from build123d import *

# Parameters (mm, degrees)
EXTRUDE_1_DEPTH     = 8
FILLET_1_R          = 20
SKETCH_5_R          = 10.5
SKETCH_5_R_2        = 6
CUT_EXTRUDE_4_DEPTH = 10
CUT_EXTRUDE_5_DEPTH = 10


with BuildPart() as part:
    # 草图1 → 凸台-拉伸1 (new body)
    with BuildSketch(Plane.XY):
        with BuildLine():
            Line((0, -10), (0, 10))
            Line((0, 10), (11.180339887, 10))
            ThreePointArc((11.180339887, 10), (-15, 0), (11.180339887, -10))
            Line((11.180339887, -10), (0, -10))
        make_face()
        with BuildLine():
            Line((11.180339887, 10), (0, 10))
            Line((0, 10), (0, -10))
            Line((0, -10), (11.180339887, -10))
            ThreePointArc((11.180339887, -10), (14.012585384, -5.352331347), (15, 0))
            ThreePointArc((15, 0), (14.012585384, 5.352331347), (11.180339887, 10))
        make_face()
        with BuildLine():
            Line((188.819660113, 10), (11.180339887, 10))
            ThreePointArc((11.180339887, 10), (14.012585384, 5.352331347), (15, 0))
            ThreePointArc((15, 0), (14.012585384, -5.352331347), (11.180339887, -10))
            Line((11.180339887, -10), (188.819660113, -10))
            ThreePointArc((188.819660113, -10), (185, 0), (188.819660113, 10))
        make_face()
        with BuildLine():
            ThreePointArc((215, 0), (205.352331347, 14.012585384), (188.819660113, 10))
            Line((188.819660113, 10), (200, 10))
            Line((200, 10), (200, -10))
            Line((200, -10), (188.819660113, -10))
            ThreePointArc((188.819660113, -10), (205.352331347, -14.012585384), (215, 0))
        make_face()
        with BuildLine():
            Line((200, 10), (188.819660113, 10))
            ThreePointArc((188.819660113, 10), (185, 0), (188.819660113, -10))
            Line((188.819660113, -10), (200, -10))
            Line((200, -10), (200, 10))
        make_face()
    extrude(amount=EXTRUDE_1_DEPTH)

    # 圆角1
    fillet_1_edges = [part.edges().sort_by_distance(p)[0] for p in [
        (11.180339887, 10, 4),
        (188.819660113, 10, 4),
        (188.819660113, -10, 4),
        (11.180339887, -10, 4),
    ]]
    fillet(fillet_1_edges, radius=FILLET_1_R)

    # 草图5 → 切除-拉伸4 (cut)
    with BuildSketch(Plane.XY.offset(8)):
        Circle(SKETCH_5_R)
        with Locations((200, 0)):
            Circle(SKETCH_5_R_2)
    extrude(amount=-CUT_EXTRUDE_4_DEPTH, mode=Mode.SUBTRACT)

    # 草图6 → 切除-拉伸5 (cut)
    with BuildSketch(Plane.XY.offset(8)):
        with BuildLine():
            ThreePointArc((31, 0), (29.535533906, -3.535533906), (26, -5))
            Line((26, -5), (62, -5))
            ThreePointArc((62, -5), (57, 0), (62, 5))
            Line((62, 5), (26, 5))
            ThreePointArc((26, 5), (29.535533906, 3.535533906), (31, 0))
        make_face()
        with BuildLine():
            ThreePointArc((26, 5), (21, 0), (26, -5))
            Line((26, -5), (26, 5))
        make_face()
        with BuildLine():
            Line((26, 5), (26, -5))
            ThreePointArc((26, -5), (29.535533906, -3.535533906), (31, 0))
            ThreePointArc((31, 0), (29.535533906, 3.535533906), (26, 5))
        make_face()
        with BuildLine():
            ThreePointArc((62, 5), (57, 0), (62, -5))
            Line((62, -5), (62, 5))
        make_face()
        with BuildLine():
            Line((62, 5), (62, -5))
            ThreePointArc((62, -5), (65.535533906, -3.535533906), (67, 0))
            ThreePointArc((67, 0), (65.535533906, 3.535533906), (62, 5))
        make_face()
        with BuildLine():
            ThreePointArc((82, 5), (77, 0), (82, -5))
            Line((82, -5), (82, 5))
        make_face()
        with BuildLine():
            Line((82, 5), (82, -5))
            ThreePointArc((82, -5), (85.535533906, -3.535533906), (87, 0))
            ThreePointArc((87, 0), (85.535533906, 3.535533906), (82, 5))
        make_face()
        with BuildLine():
            ThreePointArc((87, 0), (85.535533906, -3.535533906), (82, -5))
            Line((82, -5), (118, -5))
            ThreePointArc((118, -5), (113, 0), (118, 5))
            Line((118, 5), (82, 5))
            ThreePointArc((82, 5), (85.535533906, 3.535533906), (87, 0))
        make_face()
        with BuildLine():
            ThreePointArc((118, 5), (113, 0), (118, -5))
            Line((118, -5), (118, 5))
        make_face()
        with BuildLine():
            Line((118, 5), (118, -5))
            ThreePointArc((118, -5), (121.535533906, -3.535533906), (123, 0))
            ThreePointArc((123, 0), (121.535533906, 3.535533906), (118, 5))
        make_face()
        with BuildLine():
            ThreePointArc((138, 5), (133, 0), (138, -5))
            Line((138, -5), (138, 5))
        make_face()
        with BuildLine():
            Line((138, 5), (138, -5))
            ThreePointArc((138, -5), (141.535533906, -3.535533906), (143, 0))
            ThreePointArc((143, 0), (141.535533906, 3.535533906), (138, 5))
        make_face()
        with BuildLine():
            ThreePointArc((143, 0), (141.535533906, -3.535533906), (138, -5))
            Line((138, -5), (174, -5))
            ThreePointArc((174, -5), (169, 0), (174, 5))
            Line((174, 5), (138, 5))
            ThreePointArc((138, 5), (141.535533906, 3.535533906), (143, 0))
        make_face()
        with BuildLine():
            ThreePointArc((174, 5), (169, 0), (174, -5))
            Line((174, -5), (174, 5))
        make_face()
        with BuildLine():
            Line((174, 5), (174, -5))
            ThreePointArc((174, -5), (177.535533906, -3.535533906), (179, 0))
            ThreePointArc((179, 0), (177.535533906, 3.535533906), (174, 5))
        make_face()
    extrude(amount=-CUT_EXTRUDE_5_DEPTH, mode=Mode.SUBTRACT)


solid = part.part
CAD build for the part. Positions are in the model's coordinates, mm. A direction names the side the tool comes from. Round coordinates to 2 decimals unless told otherwise and drop trailing zeros. Order: outer loops, then holes, each group sorted by start corner. A loop starts at its lowest first (then second) coordinate and runs counter-clockwise, first axis right, second up. Notation, with made-up numbers: (17, 26.5) - (35, 26.5) arc R15 ccw to (35, 42.5) - close; hole circle Ø9 at (85, 56.25). An arc over 180 degrees is marked (long way). Return JSON: item names as keys, results as strings.
(1) Tool access for faces 4 (the face through (12.756, 10.707, 4.056)), 5 (the face through (99, -10, 4)), 6 (the face through (44, 5, 4)), 7 (the face through (98, -6, 0)): list every direction of +Z, -Z, +X, -X, +Y, -Y with a clear straight run to the whole face (end or side of a thin tool).
Answer key:
{"face 4": "+Z, -Z, +Y", "face 5": "+Z, -Z, -Y", "face 6": "+Z, -Z", "face 7": "-Z, +X, -X, +Y, -Y"}
(2) Cut at D-D (x = 71). Give the cut face in (y, z).
Answer key:
{"outline": "(-10, 0) - (10, 0) - (10, 8) - (-10, 8) - close"}
(3) Cut at A-A (x = 165). Give the cut face in (y, z), then the cut area to 3 significant figures.
Answer key:
{"outline": "(-10, 0) - (-5, 0) - (-5, 8) - (-10, 8) - close; (5, 0) - (10, 0) - (10, 8) - (5, 8) - close", "area": "80.0 mm^2"}
(4) Cut at C-C (x = 0). Give the cut face in (y, z).
Answer key:
{"outline": "(-15, 0) - (-10.5, 0) - (-10.5, 8) - (-15, 8) - close; (10.5, 0) - (15, 0) - (15, 8) - (10.5, 8) - close"}
(5) Pull direction Y, two halves, no side cores. Call faces 1 (the face through (77, 0, 4)), 2 (the face through (-15, 0, 4)), 3 (the face through (187.244, -10.707, 4.056)): +Y half, -Y half, draft (parallel to the pull), parting line (faces both ways), or undercut.
Answer key:
{"face 1": "undercut", "face 2": "parting line", "face 3": "-Y half"}
(6) Pin check, flat tips, straight feed: pin 1 Ø3 at (x, z) = (78, 3.5) entering from -Y; pin 2 Ø4 at (x, z) = (111, 4) entering from +Y; pin 3 Ø2 at (y, z) = (9, 5) entering from -X. Stop position of each tip, or through.
Answer key:
{"pin 1": "stops at y = -10", "pin 2": "stops at y = 10", "pin 3": "stops at x = -12.69"}
(7) Wall check: probe 1 along Y at (x, z) = (0, 3.75); probe 2 along Y at (x, z) = (37.5, 5); probe 3 along X at (y, z) = (5.25, 1.5). Give the ranges that are in metal, low to high. Write a range as from..to.
Answer key:
{"probe 1": "y = -15..-10.5, 10.5..15", "probe 2": "y = -10..-5, 5..10", "probe 3": "x = -14.05..-9.09, 9.09..197.1, 202.9..214.05"}
(8) Cut at B-B (z = 1.25). Give the cut face in (x, y), then the cut area to 3 significant figures.
Answer key:
{"outline": "(7.73, -12.86) arc R20 cw to (18.03, -10) - (181.97, -10) arc R20 cw to (192.27, -12.86) arc R15 ccw (long way) to (192.27, 12.86) arc R20 cw to (181.97, 10) - (18.03, 10) arc R20 cw to (7.73, 12.86) arc R15 ccw (long way) to start; hole circle Ø21 at (0, 0); hole (26, -5) - (62, -5) arc R5 ccw to (62, 5) - (26, 5) arc R5 ccw to start; hole (82, -5) - (118, -5) arc R5 ccw to (118, 5) - (82, 5) arc R5 ccw to start; hole (138, -5) - (174, -5) arc R5 ccw to (174, 5) - (138, 5) arc R5 ccw to start; hole circle Ø12 at (200, 0)", "area": "3,100 mm^2"}
